The model under review builds one solid part; all positions refer to its coordinate system, in mm. Give positions to 0.01 mm unless a question says otherwise; leave off trailing zeros. Order: outer loops, then holes, each group sorted by start corner. A loop starts at its lowest first (then second) coordinate and runs counter-clockwise, first axis right, second up.
Autodesk Inventor part; units mm, degrees
ref_plane "YZ Plane" through (0, 0, 0) normal (1, 0, 0) x (0, 1, 0)
ref_plane "XZ Plane" through (0, 0, 0) normal (0, 1, 0) x (-1, 0, 0)
ref_plane "XY Plane" through (0, 0, 0) normal (0, 0, 1) x (1, 0, 0)
sketch "Sketch1" plane through (0, 0, 0) normal (0, 1, 0) x (-1, 0, 0)
  line L0 (93.9, 88.9) -> (-93.9, 88.9)
  line L1 (-93.9, 88.9) -> (-93.9, -88.9)
  line L2 (-93.9, -88.9) -> (93.9, -88.9)
  line L3 (93.9, -88.9) -> (93.9, 88.9)
  line L4 (93.9, 88.9) -> (-93.9, -88.9) construction
  line L5 (-93.9, 88.9) -> (93.9, -88.9) construction
  point P0 (0, 0)
  dimension "d0" = 187.8
  dimension "d1" = 177.8
extrude "Extrusion1" add sketch "Sketch1" along normal blind 6.35
sketch "Sketch3" plane through (0, 6.35, 0) normal (0, 1, 0) x (1, 0, 0)
  line L0 (-93.9, 88.9) -> (-93.9, -88.9)
  line L1 (93.9, 88.9) -> (-93.9, 88.9)
  line L2 (-86.5034, 24.275) -> (-86.5034, -25.725) construction
  line L3 (-86.5034, -25.725) -> (-38.5034, -25.725) construction
  line L4 (-38.5034, -25.725) -> (-38.5034, 24.275) construction
  line L5 (-38.5034, 24.275) -> (-86.5034, 24.275) construction
  line L6 (38.5034, 24.275) -> (38.5034, -25.725) construction
  line L7 (38.5034, -25.725) -> (86.5034, -25.725) construction
  line L8 (86.5034, -25.725) -> (86.5034, 24.275) construction
  line L9 (86.5034, 24.275) -> (38.5034, 24.275) construction
  line L10 (-86.5034, -35.725) -> (-86.5034, -85.725) construction
  line L11 (-86.5034, -85.725) -> (-38.5034, -85.725) construction
  line L12 (-38.5034, -85.725) -> (-38.5034, -35.725) construction
  line L13 (-38.5034, -35.725) -> (-86.5034, -35.725) construction
  line L14 (38.5034, -35.725) -> (38.5034, -85.725) construction
  line L15 (38.5034, -85.725) -> (86.5034, -85.725) construction
  line L16 (86.5034, -85.725) -> (86.5034, -35.725) construction
  line L17 (86.5034, -35.725) -> (38.5034, -35.725) construction
  line L18 (-24, -13.225) -> (24, -13.225) construction
  line L19 (24, -13.225) -> (24, -48.225) construction
  line L20 (24, -48.225) -> (-24, -48.225) construction
  line L21 (-24, -48.225) -> (-24, -13.225) construction
  line L22 (93.9, -88.9) -> (93.9, 88.9)
  line L23 (-93.9, -88.9) -> (93.9, -88.9)
  point P0 (-133.35, 152.4)
  point P1 (-152.4, 133.35)
  point P2 (-152.4, -133.35)
  point P3 (133.35, 152.4)
  point P4 (0, -30.725)
  point P5 (-80.0034, 16.775)
  point P6 (-45.0034, 16.775)
  point P7 (-80.0034, -18.225)
  point P8 (-45.0034, -18.225)
  point P9 (45.0034, 16.775)
  point P10 (80.0034, 16.775)
  point P11 (45.0034, -18.225)
  point P12 (80.0034, -18.225)
  point P13 (-80.0034, -43.225)
  point P14 (-45.0034, -43.225)
  point P15 (-80.0034, -78.225)
  point P16 (-45.0034, -78.225)
  point P17 (45.0034, -43.225)
  point P18 (80.0034, -43.225)
  point P19 (45.0034, -78.225)
  point P20 (80.0034, -78.225)
  point P21 (0, -13.225)
  point P22 (62.5034, -30.725)
  point P23 (24, -30.725)
  point P24 (62.5034, 24.275)
  point P25 (-19, -19.725)
  point P26 (19, -19.725)
  point P27 (-19, -41.725)
  point P28 (19, -41.725)
  point P29 (-93.9, 88.9)
  dimension "d27" = 35
  dimension "d30" = 35
  dimension "d33" = 48
  dimension "d34" = 50
  dimension "d35" = 6.5
  dimension "d36" = 6.5
  dimension "d37" = 7.5
  dimension "d38" = 7.5
  dimension "d42" = 125.0068
  dimension "d45" = 60
  dimension "d50" = 48
  dimension "d51" = 35
  dimension "d52" = 5
  dimension "d53" = 6.5
  dimension "d56" = 38
  dimension "d59" = 22
  dimension "d78" = 14.5034
  dimension "d79" = 14.5034
  dimension "d80" = 10
  dimension "d81" = 5
  dimension "d82" = 173.0068
  dimension "d83" = 110
  dimension "d84" = 102.125
  dimension "d85" = 69.9
  dimension "d115" = 7.3966
  dimension "d116" = 7.3966
  dimension "d117" = 3.175
hole "Hole4" at (-80.0034, 6.35, 18.225) at (-80.0034, 6.35, -16.775) at (-80.0034, 6.35, 43.225) at (-80.0034, 6.35, 78.225) at (-45.0034, 6.35, 43.225) at (-45.0034, 6.35, 78.225) at (-45.0034, 6.35, 18.225) at (-45.0034, 6.35, -16.775) at (80.0034, 6.35, -16.775) at (80.0034, 6.35, 18.225) at (80.0034, 6.35, 43.225) at (80.0034, 6.35, 78.225) at (45.0034, 6.35, 78.225) at (45.0034, 6.35, 43.225) at (45.0034, 6.35, 18.225) at (45.0034, 6.35, -16.775) direction (0, -1, 0) diameter 6.6 end through all
hole "Hole5" at (-19, 6.35, 19.725) at (19, 6.35, 19.725) at (-19, 6.35, 41.725) at (19, 6.35, 41.725) direction (0, -1, 0) diameter 5.5 end through all
hole "Hole6" at (-80.0034, 6.35, -16.775) at (-45.0034, 6.35, -16.775) at (-45.0034, 6.35, 18.225) at (-80.0034, 6.35, 18.225) at (-80.0034, 6.35, 43.225) at (-45.0034, 6.35, 43.225) at (-45.0034, 6.35, 78.225) at (-80.0034, 6.35, 78.225) at (80.0034, 6.35, 78.225) at (80.0034, 6.35, 43.225) at (80.0034, 6.35, -16.775) at (80.0034, 6.35, 18.225) at (45.0034, 6.35, -16.775) at (45.0034, 6.35, 18.225) at (45.0034, 6.35, 78.225) at (45.0034, 6.35, 43.225) direction (0, -1, 0) diameter 10.6 depth 3.3
hole "Hole7" at (-19, 6.35, 19.725) at (19, 6.35, 19.725) at (19, 6.35, 41.725) at (-19, 6.35, 41.725) direction (0, -1, 0) diameter 9.6 depth 2.75
sketch "Sketch6" plane through (0, 6.35, 0) normal (0, 1, 0) x (1, 0, 0)
  line L0 (-93.9, -88.9) -> (93.9, -88.9)
  line L1 (-28.194, -104.775) -> (28.194, -104.775)
  line L2 (28.194, -104.775) -> (28.194, -73.025)
  line L3 (28.194, -73.025) -> (-28.194, -73.025)
  line L4 (-28.194, -73.025) -> (-28.194, -104.775)
  line L5 (-28.194, -104.775) -> (28.194, -73.025) construction
  line L6 (28.194, -104.775) -> (-28.194, -73.025) construction
  point P0 (0, 0)
  point P1 (0, -88.9)
  dimension "d118" = 56.388
  dimension "d119" = 31.75
extrude "Extrusion2" cut sketch "Sketch6" against normal blind 25.4
equation "\"d78\" = d79"
equation "\"d116\" = d115"
equation "\"d91\" = d59"
equation "\"d98\" = d59"
properties part number "mic6_plate"
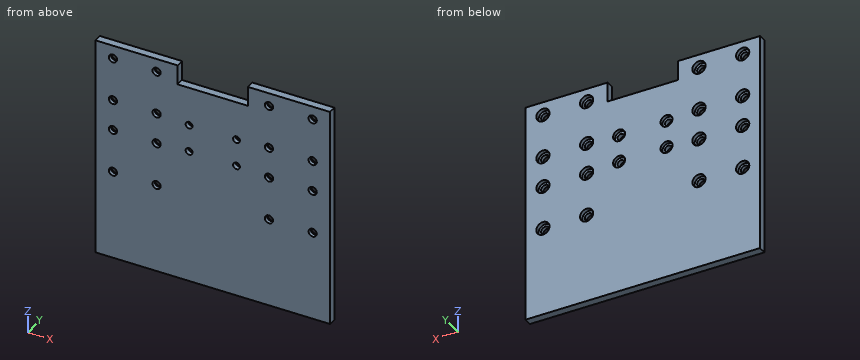
Item 1: Take a section at A-A (x = 19). Give the boundary of the cut face in (y, z) (3 decimals), and give its area (3 significant figures).
Values found:
outline: (0, -88.9) - (6.35, -88.9) - (6.35, 14.925) - (3.6, 14.925) - (3.6, 16.975) - (0, 16.975) - close; (0, 22.475) - (3.6, 22.475) - (3.6, 24.525) - (6.35, 24.525) - (6.35, 36.925) - (3.6, 36.925) - (3.6, 38.975) - (0, 38.975) - close; (0, 44.475) - (3.6, 44.475) - (3.6, 46.525) - (6.35, 46.525) - (6.35, 73.025) - (0, 73.025) - close
area: 936 mm2
Item 2: Clearance check with flat-ended pins moving along their axes: pin 1 Ø1 at (x, y) = (23, 5.5) entering from +Z (3 decimals); pin 2 Ø6 at (x, z) = (-80, -16.77) entering from +Y; pin 3 Ø8.5 at (x, z) = (-80, 78.22) entering from +Y. State where each tip first meets the part, or that it passes through.
Values found:
pin 1: stops at z = 73.025
pin 2: passes through
pin 3: stops at y = 3.05
Item 3: For line 1 (Z direction, x = 19, y = 3.25) (3 decimals); line 2 (Z direction, x = 48.5, y = 4); line 3 (Z direction, x = 0.5, y = 0.75) (3 decimals), list the stretches that pass through material, from the lowest coordinate up.
Values found:
line 1: z = -88.9 to 16.975, 22.475 to 38.975, 44.475 to 73.025
line 2: z = -88.9 to -20.76, -12.79 to 14.24, 22.21 to 39.24, 47.21 to 74.24, 82.21 to 88.9
line 3: z = -88.9 to 73.025
Item 4: Take a section at B-B (x = -12). Give the boundary of the cut face in (y, z) (3 decimals), and give its area (3 significant figures).
Values found:
outline: (0, -88.9) - (6.35, -88.9) - (6.35, 73.025) - (0, 73.025) - close
area: 1,030 mm2
